Geometry: final body of the model. Coordinates: model frame, mm. Give positions to 0.01 mm unless a question says otherwise; leave off trailing zeros. Order: outer loops, then holes, each group sorted by start corner. A loop starts at its lowest first (then second) coordinate and runs counter-clockwise, first axis right, second up. Notation, with made-up numbers: M 32.5,5 L 79.5,5 A23 ccw 79.5,29 Z; hole C -19.75,-34.5 d4. An arc over 180 degrees is marked long. Write item = value, one per line. Start each with the question number.
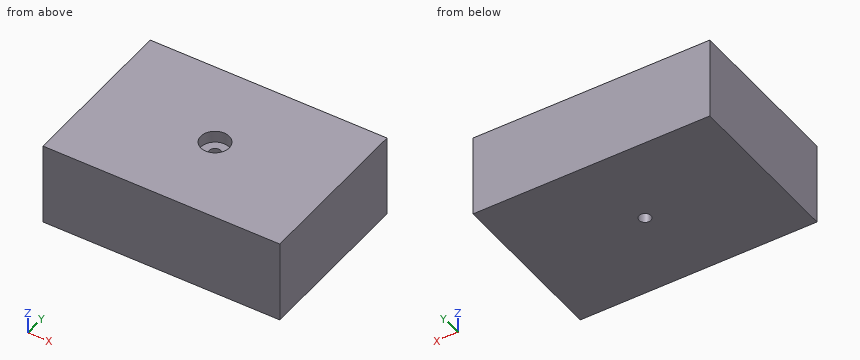
from build123d import *

# Parameters (mm, degrees)
F0_W           = 100
F0_H           = 70
F1_DEPTH       = 17.5
F3_D           = 5
F3_CBORE_D     = 12
F3_CBORE_DEPTH = 5


with BuildPart() as f1:
    # F0 (on Top) → F1 (new body, symmetric)
    with BuildSketch(Plane.XY):
        Rectangle(F0_W, F0_H)
    extrude(amount=F1_DEPTH, both=True)

    # F3 (through all)
    with Locations(Plane.XY.offset(17.5)):
        with Locations((0, 0)):
            CounterBoreHole(F3_D / 2, F3_CBORE_D / 2, F3_CBORE_DEPTH)


solid = f1.part
1) Cut plane B-B (y = 0). Return loops of the section in (x, z).
2) Cut plane A-A (x = 0). Return loops of the section in (y, z), plus the area to 3 significant figures.
3) Pin query (flat end, axial travel): pin 1 Ø6 at (x, y) = (1.5, 1.5) entering from +Z. Return the tip coordinate at first contact, or that it passes through.
4) Ray query, L1, parallel to Y at x = 0, z = 4; L2, parallel to Y at x = 0, z = 16; L3, parallel to X at y = 0.5, z = -11.5. Return the intervals inside material, ascending.
Reply:
q1.outline = M -50,-17.5 L -2.5,-17.5 L -2.5,12.5 L -6,12.5 L -6,17.5 L -50,17.5 Z; M 2.5,-17.5 L 50,-17.5 L 50,17.5 L 6,17.5 L 6,12.5 L 2.5,12.5 Z
q2.outline = M -35,-17.5 L -2.5,-17.5 L -2.5,12.5 L -6,12.5 L -6,17.5 L -35,17.5 Z; M 2.5,-17.5 L 35,-17.5 L 35,17.5 L 6,17.5 L 6,12.5 L 2.5,12.5 Z
q2.area = 2,240 mm²
q3.pin_1 = 12.5
q4.L1 = -35 to -2.5, 2.5 to 35
q4.L2 = -35 to -6, 6 to 35
q4.L3 = -50 to -2.45, 2.45 to 50
